Verification items for the finished model (mm, model axes). Face numbers are marked on the shaded views. Round coordinates to 2 decimals unless told otherwise and drop trailing zeros. Write each loop counter-clockwise with the first axis right and the second up, starting at its lowest first coordinate (ties: lowest second). Pieces come first, ordered by that corner, then holes. Notation, with made-up numbers: (1, -29) -> (27, -29) arc R7 ccw to (27, -23) -> close; hole circle Ø5 at (-19, 62). An arc over 180 degrees is marked (long way). Answer as a JSON object with one key per item and string values. Group by question number.
(1) Sectioned sample at B-B on x = 99.06. Record the cut outline in (y, z) (3 decimals).
(2) Scan lines: L1, parallel to X at y = -4.75, z = 2.25; L2, parallel to X at y = -10, z = 0.5; L3, parallel to X at y = -2.5, z = 4.25. Record each from-to range of solid material in increasing order. Write a range as from..to.
(3) Sectioned sample at C-C on z = 7. Record the cut outline in (x, y).
(4) Gauge pin test, flat ends, axial feed: pin 1 Ø1 at (y, z) = (-2.5, 7) entering from -X; pin 2 Ø4 at (y, z) = (-5, 5) entering from -X; pin 3 Ø2 at (y, z) = (-10.5, 6.5) entering from +X. Record the tip position at first contact, or that the pin passes through.
(5) Draft check along X on the marked faces 1, 2 and 3. Enter one of: released by +X, released by -X, zero draft, split by the parting line, or undercut.
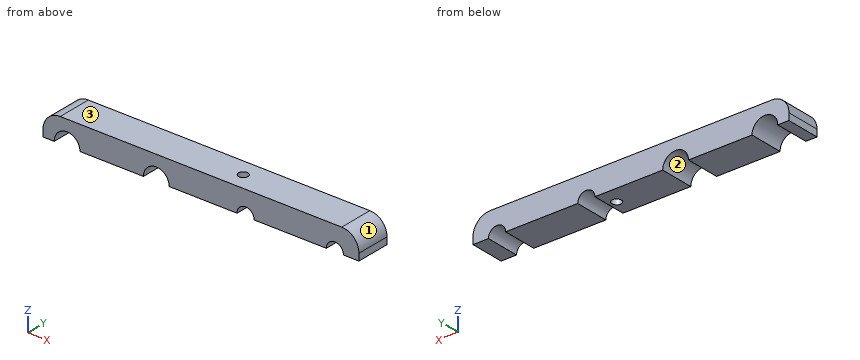
```python
from build123d import *

# Parameters (mm, degrees)
F1_DEPTH = 12.7
F2_R     = 1.7526
F3_DEPTH = 25.4


with BuildPart() as f1:
    # F0 (on Front) → F1 (new body)
    with BuildSketch(Plane.XZ):
        with BuildLine():
            ThreePointArc((-4.7625, 0), (0, 4.7625), (4.7625, 0))
            Line((4.7625, 0), (28.2575, 0))
            ThreePointArc((28.2575, 0), (33.02, 4.7625), (37.7825, 0))
            Line((37.7825, 0), (62.865, 0))
            ThreePointArc((62.865, 0), (66.04, 3.175), (69.215, 0))
            Line((69.215, 0), (95.885, 0))
            ThreePointArc((95.885, 0), (99.06, 3.175), (102.235, 0))
            Line((102.235, 0), (107.95, 0))
            Line((107.95, 0), (107.95, 2.54))
            ThreePointArc((107.95, 2.54), (106.090128, 7.030128), (101.6, 8.89))
            Line((101.6, 8.89), (-2.54, 8.89))
            ThreePointArc((-2.54, 8.89), (-7.030128, 7.030128), (-8.89, 2.54))
            Line((-8.89, 2.54), (-8.89, 0))
            Line((-8.89, 0), (-4.7625, 0))
        make_face()
    extrude(amount=F1_DEPTH)

    # F2 (on face) → F3 (cut)
    with BuildSketch(Plane.XY.offset(8.89)):
        with Locations((60.0075, -6.35)):
            Circle(F2_R)
    extrude(amount=-F3_DEPTH, mode=Mode.SUBTRACT)


solid = f1.part
```
Computed values:
{
 "1": {"outline": "(-12.7, 3.175) -> (0, 3.175) -> (0, 8.89) -> (-12.7, 8.89) -> close"},
 "2": {"L1": "-8.89..-4.2, 4.2..28.82, 37.22..59.29, 60.72..63.8, 68.28..96.82, 101.3..107.95", "L2": "-8.89..-4.74, 4.74..28.28, 37.76..62.9, 69.18..95.92, 102.2..107.95", "L3": "-8.66..-2.15, 2.15..30.87, 35.17..107.72"},
 "3": {"outline": "(-7.06, -12.7) -> (106.12, -12.7) -> (106.12, 0) -> (-7.06, 0) -> close; hole circle Ø3.51 at (60.01, -6.35)"},
 "4": {"pin 1": "x = -7.5", "pin 2": "x = -8.87", "pin 3": "x = 107.22"},
 "5": {"face 1": "released by +X", "face 2": "undercut", "face 3": "zero draft"}
}
